Here's the drawing with two shaded views (mm, measured from the low corner). I have some questions. A direction names the side the tool comes from. Round coordinates to 2 decimals unless told otherwise and drop trailing zeros. Loops run counter-clockwise (first coordinate to the right, second up) from the corner with the lowest first, then second, coordinate; pieces in that order, holes last. Notation, with made-up numbers: (71.5, 30) - (115.5, 30) arc R23 ccw to (115.5, 64) - close; hole circle Ø11 at (52, -17.75). An arc over 180 degrees is marked (long way). Answer as CSV lines item,"result".
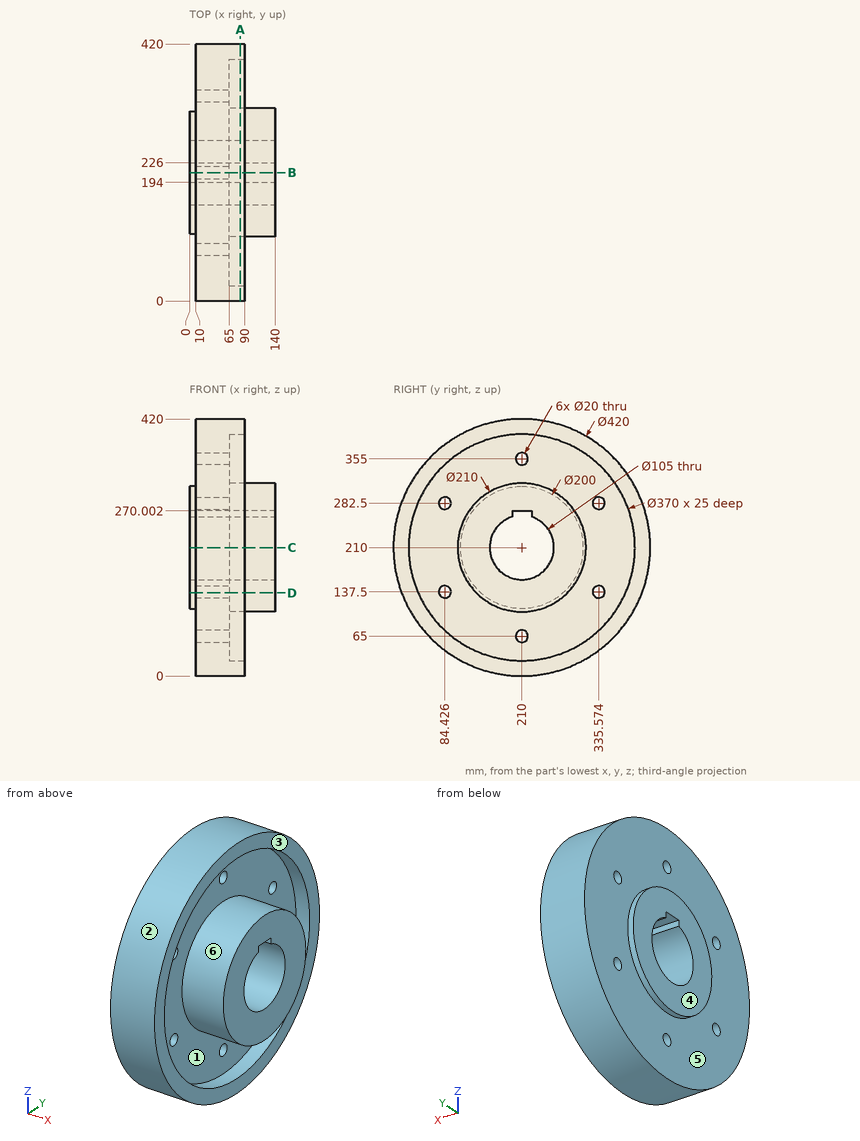
Q1. We'd pull the mould along Z, two halves only. Please class the marked faces 1, 2 and 3: pulls with the +Z half, pulls with the -Z half, needs draft (parallel to the pull), parting line crosses it, or undercut.
Checks:
face 1,"undercut"
face 2,"parting line crosses it"
face 3,"needs draft"
Q2. Imagine slicing it at C-C (z = 210). Write out the boundary of the cut face in (x, y), then the cut area to 3 significant figures.
Checks:
outline,"(0, 110) - (10, 110) - (10, 0) - (90, 0) - (90, 25) - (65, 25) - (65, 105) - (140, 105) - (140, 157.5) - (0, 157.5) - close; (0, 262.5) - (140, 262.5) - (140, 315) - (65, 315) - (65, 395) - (90, 395) - (90, 420) - (10, 420) - (10, 310) - (0, 310) - close"
area,"27,400 mm²"
Q3. Imagine slicing it at A-A (x = 83). Write out the boundary of the cut face in (y, z), then the cut area to 3 significant figures.
Checks:
outline,"circle Ø420 at (210, 210); circle Ø210 at (210, 210); hole circle Ø370 at (210, 210); hole (194, 260) arc R52.5 ccw (long way) to (226, 260) - (226, 270) - (194, 270) - close"
area,"56,700 mm²"
Q4. If I drill on line 1 along Z through (x, y) = (71.5, 210); line 2 along Z through (x, y) = (83.5, 237) (1 decimal); line 3 along Z through (x, y) = (68.5, 275.5) (1 decimal), over which ranges is the centre line in solid material (lowest first)? Write a range as [from, to].
Checks:
line 1,"[0, 25], [105, 157.5], [270, 315], [395, 420]"
line 2,"[1.7, 27], [108.5, 165], [255, 311.5], [393, 418.3]"
line 3,"[10.5, 37], [127.9, 292.1], [383, 409.5]"
Q5. Imagine slicing it at B-B (y = 210). Write out the boundary of the cut face in (x, z).
Checks:
outline,"(0, 110) - (10, 110) - (10, 75) - (65, 75) - (65, 105) - (140, 105) - (140, 157.5) - (0, 157.5) - close; (0, 270) - (140, 270) - (140, 315) - (65, 315) - (65, 345) - (10, 345) - (10, 310) - (0, 310) - close; (10, 0) - (90, 0) - (90, 25) - (65, 25) - (65, 55) - (10, 55) - close; (10, 365) - (65, 365) - (65, 395) - (90, 395) - (90, 420) - (10, 420) - close"
Q6. Imagine slicing it at D-D (z = 136). Write out the boundary of the cut face in (x, y) (1 decimal), then the cut area to 3 significant figures.
Checks:
outline,"(0, 142.7) - (10, 142.7) - (10, 94.3) - (65, 94.3) - (65, 135.5) - (140, 135.5) - (140, 284.5) - (65, 284.5) - (65, 325.7) - (10, 325.7) - (10, 277.3) - (0, 277.3) - close; (10, 13.5) - (90, 13.5) - (90, 40.4) - (65, 40.4) - (65, 74.5) - (10, 74.5) - close; (10, 345.5) - (65, 345.5) - (65, 379.6) - (90, 379.6) - (90, 406.5) - (10, 406.5) - close"
area,"33,300 mm²"
Q7. On a 3-axis mill with a long thin cutter (end or side, diameter ignored), from which of +Z, -Z, +X, -X, +Y, -Y can I reach the whole of each face in a straight line? I mean the marked faces 4, 5 and 6. Say none if no direction works.
Checks:
face 4,"+Z, -Z, -X, +Y, -Y"
face 5,"-X"
face 6,"+X"
Q8. I'm going to push flat-ended pins straight in: pin 1 Ø10 at (x, z) = (42, 64) entering from -Y (1 decimal); pin 2 Ø5 at (x, z) = (48, 264) entering from -Y; pin 3 Ø6 at (y, z) = (298.5, 59.5) entering from -X. Where does each tip first touch, or does it pass through?
Checks:
pin 1,"y = 54.4"
pin 2,"y = 6.41"
pin 3,"x = 10"
